Design review of the part built by this model. Coordinates are the model's own, in mm. Round coordinates to 2 decimals unless told otherwise and drop trailing zeros. Loops run counter-clockwise (first coordinate to the right, second up) from the corner with the lowest first, then second, coordinate; pieces in that order, holes last. Notation, with made-up numbers: (82.25, 5) - (136.25, 5) arc R14 ccw to (136.25, 9) - close; hole circle Ø2 at (-13, -9.5). An arc over 180 degrees is marked (long way). Return JSON: item names as keys, results as strings. Group by question number.
from build123d import *

# Parameters (mm, degrees)
SKETCH_1_W          = 11
SKETCH_1_H          = 15
EXTRUDE_1_DEPTH     = 1.5
SKETCH_2_R          = 2.5
CUT_EXTRUDE_1_DEPTH = 1.5
CHAMFER_1_SIZE      = 0.2
CHAMFER_2_SIZE      = 0.2


with BuildPart() as part:
    # ｽｹｯﾁ1 → ﾎﾞｽ - 押し出し1 (new body)
    with BuildSketch(Plane(origin=(0, 0, 0), x_dir=(1, 0, 0), z_dir=(0, 1, 0))):
        Rectangle(SKETCH_1_W, SKETCH_1_H)
    extrude(amount=EXTRUDE_1_DEPTH)

    # ｽｹｯﾁ2 → ｶｯﾄ - 押し出し1 (cut)
    with BuildSketch(Plane(origin=(0, 1.5, 0), x_dir=(1, 0, 0), z_dir=(0, 1, 0))):
        with Locations(Location((0, 0, 0), (0, 0, 270))):
            Circle(SKETCH_2_R)
    extrude(amount=-CUT_EXTRUDE_1_DEPTH, mode=Mode.SUBTRACT)

    # 面取り1
    chamfer_1_edges = [part.edges().sort_by_distance(p)[0] for p in [
        (-5.5, 1.5, 0),
        (0, 1.5, 7.5),
        (5.5, 1.5, 0),
        (0, 1.5, -7.5),
    ]]
    chamfer(chamfer_1_edges, length=CHAMFER_1_SIZE)

    # 面取り2
    chamfer_2_edges = [part.edges().sort_by_distance(p)[0] for p in [
        (0, 0, 7.5),
        (-5.5, 0, 0),
        (0, 0, -7.5),
        (5.5, 0, 0),
    ]]
    chamfer(chamfer_2_edges, length=CHAMFER_2_SIZE)


solid = part.part
Q1. Add section B-B, the plane z = 0. State the section outline as (x, y) points.
Q2. For line 1 (X direction, y = 1, z = 0); line 2 (X direction, y = 0.5, z = 1.75); line 3 (Z direction, x = 2.25, y = 1), list the stretches that pass through material, from the lowest coordinate up.
Q3. Add section A-A, the plane x = 2. State the section outline as (y, z) points, plus the area to 3 significant figures.
Q4. Add section C-C, the plane y = 0.7. State the section outline as (x, z) points.
Evaluation:
{
 "1": {"outline": "(-5.5, 0.2) - (-5.3, 0) - (-2.5, 0) - (-2.5, 1.5) - (-5.3, 1.5) - (-5.5, 1.3) - close; (2.5, 0) - (5.3, 0) - (5.5, 0.2) - (5.5, 1.3) - (5.3, 1.5) - (2.5, 1.5) - close"},
 "2": {"line 1": "-5.5 to -2.5, 2.5 to 5.5", "line 2": "-5.5 to -1.79, 1.79 to 5.5", "line 3": "-7.5 to -1.09, 1.09 to 7.5"},
 "3": {"outline": "(0, -7.3) - (0.2, -7.5) - (1.3, -7.5) - (1.5, -7.3) - (1.5, -1.5) - (0, -1.5) - close; (0, 1.5) - (1.5, 1.5) - (1.5, 7.3) - (1.3, 7.5) - (0.2, 7.5) - (0, 7.3) - close", "area": "17.9 mm²"},
 "4": {"outline": "(-5.5, -7.5) - (5.5, -7.5) - (5.5, 7.5) - (-5.5, 7.5) - close; hole circle Ø5 at (0, 0)"}
}
